Geometry: final body of the model. Coordinates: model frame, mm. Give positions to 0.01 mm unless a question says otherwise; leave off trailing zeros. Write each loop counter-clockwise with the first axis right and the second up, starting at its lowest first coordinate (ties: lowest second). Pieces come first, ordered by that corner, then holes.
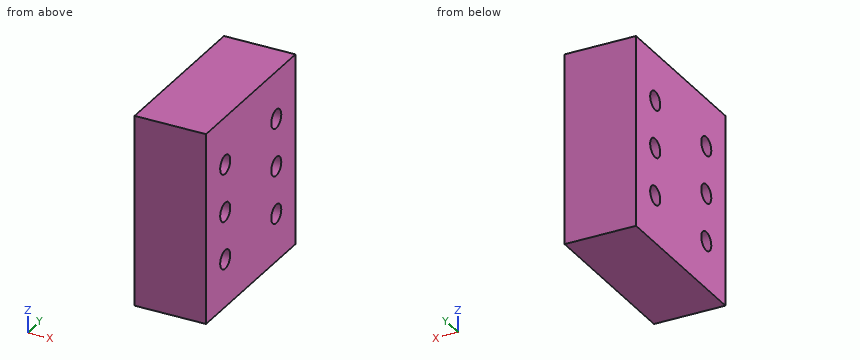
from build123d import *

# Parameters (mm, degrees)
SKETCH1_W           = 19.05
SKETCH1_H           = 44.45
BOSS_EXTRUDE1_DEPTH = 50.8
SKETCH2_R           = 2.4892
CUT_EXTRUDE1_DEPTH  = 71.138042459


with BuildPart() as part:
    # Sketch1 → Boss-Extrude1 (new body)
    with BuildSketch(Plane.XY):
        with Locations((9.525, 22.225)):
            Rectangle(SKETCH1_W, SKETCH1_H)
    extrude(amount=BOSS_EXTRUDE1_DEPTH)

    # Sketch2 → Cut-Extrude1 (cut, through all)
    with BuildSketch(Plane(origin=(19.05, 0, 0), x_dir=(0, 0, -1), z_dir=(1, 0, 0))):
        with Locations(Location((-38.1, 9.525, 0), (0, 0, 90))):
            Circle(SKETCH2_R)
        with Locations(Location((-25.4, 9.525, 0), (0, 0, 90))):
            Circle(SKETCH2_R)
        with Locations(Location((-12.7, 9.525, 0), (0, 0, 90))):
            Circle(SKETCH2_R)
        with Locations(Location((-38.1, 34.925, 0), (0, 0, 90))):
            Circle(SKETCH2_R)
        with Locations(Location((-25.4, 34.925, 0), (0, 0, 90))):
            Circle(SKETCH2_R)
        with Locations(Location((-12.7, 34.925, 0), (0, 0, 90))):
            Circle(SKETCH2_R)
    extrude(amount=-CUT_EXTRUDE1_DEPTH, mode=Mode.SUBTRACT)


solid = part.part
Q1. Pin query (flat end, axial travel): P1, Ø8, axis at y = 34.925, z = 25.4, coming from the +X side; P2, Ø4.5, axis at y = 9.525, z = 25.4, coming from the +X side. Return the tip coordinate at first contact, or that it passes through.
Filled sheet:
P1: stops at x = 19.05
P2: passes through
Q2. Section D-D on z = 36.5. Output: boundary loops of the cut face in (x, y), plus the area to 3 significant figures.
Filled sheet:
outline: (0, 0) - (19.05, 0) - (19.05, 7.62) - (0, 7.62) - close; (0, 11.43) - (19.05, 11.43) - (19.05, 33.02) - (0, 33.02) - close; (0, 36.83) - (19.05, 36.83) - (19.05, 44.45) - (0, 44.45) - close
area: 701 mm2
Q3. Section C-C on y = 8.5. Output: boundary loops of the cut face in (x, z), plus the area to 3 significant figures.
Filled sheet:
outline: (0, 0) - (19.05, 0) - (19.05, 10.43) - (0, 10.43) - close; (0, 14.97) - (19.05, 14.97) - (19.05, 23.13) - (0, 23.13) - close; (0, 27.67) - (19.05, 27.67) - (19.05, 35.83) - (0, 35.83) - close; (0, 40.37) - (19.05, 40.37) - (19.05, 50.8) - (0, 50.8) - close
area: 708 mm2
Q4. Section A-A on z = 25.4. Output: boundary loops of the cut face in (x, y), plus the area to 3 significant figures.
Filled sheet:
outline: (0, 0) - (19.05, 0) - (19.05, 7.04) - (0, 7.04) - close; (0, 12.01) - (19.05, 12.01) - (19.05, 32.44) - (0, 32.44) - close; (0, 37.41) - (19.05, 37.41) - (19.05, 44.45) - (0, 44.45) - close
area: 657 mm2
Q5. Section B-B on x = 4.25. Output: boundary loops of the cut face in (y, z) (3 decimals).
Filled sheet:
outline: (0, 0) - (44.45, 0) - (44.45, 50.8) - (0, 50.8) - close; hole circle Ø4.978 at (9.525, 12.7); hole circle Ø4.978 at (9.525, 25.4); hole circle Ø4.978 at (9.525, 38.1); hole circle Ø4.978 at (34.925, 12.7); hole circle Ø4.978 at (34.925, 25.4); hole circle Ø4.978 at (34.925, 38.1)
Q6. Ray query, line 1 along Z through (x, y) = (5.25, 35); line 2 along Z through (x, y) = (11.75, 10); line 3 along Y through (x, z) = (5, 23.5). Return the intervals inside material, ascending.
Filled sheet:
line 1: z = 0 to 10.21, 15.19 to 22.91, 27.89 to 35.61, 40.59 to 50.8
line 2: z = 0 to 10.26, 15.14 to 22.96, 27.84 to 35.66, 40.54 to 50.8
line 3: y = 0 to 7.92, 11.13 to 33.32, 36.53 to 44.45
